The model under review builds one solid part; all positions refer to its coordinate system, in mm. A direction names the side the tool comes from. Give positions to 0.01 mm unless a question says otherwise; leave off trailing zeros. Order: outer loops, then holes, each group sorted by start corner. A loop starts at its lowest first (then second) coordinate and runs counter-clockwise, first axis right, second up. Notation, with made-up numbers: (48.5, -38.5) - (101.5, -38.5) arc R30 ccw to (101.5, -1.5) - close; hole circle Ø7 at (11, -26.75). An arc over 180 degrees is marked (long way). Answer as CSV lines item,"result". Start each with the question number.
Autodesk Fusion 360 part; units mm, degrees
sketch "Sketch1" plane through (0, 0, 0) normal (0, 0, 1) x (1, 0, 0)
  circle A0 centre (0, 0) radius 62
  circle A1 centre (0, 0) radius 45
  circle A2 centre (0, 0) radius 3
  dimension "d1" = 124
  dimension "d5" = 90
  dimension "d14" = 6
extrude "Extrude1" add sketch "Sketch1" along normal blind 30 contours A0 | A1 | A2
fillet "Fillet1" radius 10 2 edges at (-57.8043, -22.4202, 30) (-57.8043, -22.4202, 0)
sketch "Sketch4" plane through (0, 0, 0) normal (0, 0, -1) x (1, 0, 0)
  circle A0 centre (0, 0) radius 52
  line L0 (6.9152, -1.8529) -> (5.0623, 5.0623)
  line L1 (5.0623, 5.0623) -> (-1.8529, 6.9152)
  line L2 (-1.8529, 6.9152) -> (-6.9152, 1.8529)
  line L3 (-6.9152, 1.8529) -> (-5.0623, -5.0623)
  line L4 (-5.0623, -5.0623) -> (1.8529, -6.9152)
  line L5 (1.8529, -6.9152) -> (6.9152, -1.8529)
  dimension "d16" = 12.4
extrude "Extrude5" cut sketch "Sketch4" against normal blind 22 contours L0 L1 L2 L3 L4 L5
extrude "Extrude2" cut sketch "Sketch1" along normal blind 5 contours A1 | A2
sketch "Sketch3" plane through (0, 0, 30) normal (0, 0, 1) x (-1, 0, 0)
  circle A0 centre (0, 0) radius 52
  circle A1 centre (0, 0) radius 45
  dimension "d9" = 90
extrude "Extrude3" cut sketch "Sketch3" against normal blind 5 contours A1
fillet "Fillet2" radius 2.5 1 edges at (41.9547, -16.2727, 30)
fillet "Fillet3" radius 2.5 1 edges at (-41.9547, -16.2727, 0)
extrude "Extrude4" cut sketch "Sketch1" along normal through all contours A2
Item 1: Clearance check with flat-ended pins moving along their axes: pin 1 (12 mm diameter, centred on x = 3, z = 20.5, fed in from +Y); pin 2 (4 mm diameter, centred on y = 49, z = 22.5, fed in from -X); pin 3 (15 mm diameter, centred on x = -3, y = 0, fed in from -Z). State where each tip first meets the part, or that it passes through.
Item 2: For line 1 along Z through (x, y) = (-42, -31); line 2 along Z through (x, y) = (-41, -9); line 3 along X through (y, z) = (31, 3.25), list the stretches that pass through material, from the lowest coordinate up.
Item 3: Machinability: for faces 4 (the face through (-20.765, 39.923, 26.268)), 5 (the face through (-3, 0, 23)), 6 (the face through (-1, -9, 5)), which of the approach directions +Z, -Z, +X, -X, +Y, -Y give a long, thin tool a straight path to every point of the face, cutting with its end or side? Answer none if there is none.
Item 4: Mouldability with a two-part tool opening along X and no side actions: class faces 1 (the face through (23, -42, 30)), 2 (the face through (4.35, 4.42, 13.38)), 3 (the face through (-8.071, -61.472, 14.93)) as released by +X, released by -X, zero draft, split by the parting line, or undercut.
Item 5: Take a section at A-A on y = 0. Write out the cut boundary in (x, z).
Data:
1,pin 1,"stops at y = 62"
1,pin 2,"stops at x = -40.05"
1,pin 3,"stops at z = 5"
2,line 1,"z = 0 to 30"
2,line 2,"z = 5 to 25"
2,line 3,"x = -50.64 to -32.62, 32.62 to 50.64"
3,face 4,"+Z"
3,face 5,"+Z, -Z"
3,face 6,"-Z"
4,face 1,"zero draft"
4,face 2,"undercut"
4,face 3,"split by the parting line"
5,outline,"(-62, 10) arc R10 ccw to (-52, 0) - (-47.5, 0) arc R2.5 ccw to (-45, 2.5) - (-45, 5) - (-6.42, 5) - (-6.42, 22) - (-3, 22) - (-3, 25) - (-45, 25) - (-45, 27.5) arc R2.5 ccw to (-47.5, 30) - (-52, 30) arc R10 ccw to (-62, 20) - close; (3, 22) - (6.42, 22) - (6.42, 5) - (45, 5) - (45, 2.5) arc R2.5 ccw to (47.5, 0) - (52, 0) arc R10 ccw to (62, 10) - (62, 20) arc R10 ccw to (52, 30) - (47.5, 30) arc R2.5 ccw to (45, 27.5) - (45, 25) - (3, 25) - close"
